Build history of the part. All positions in model axes, mm. A direction names the side the tool comes from. Coordinates: 2 decimals unless noted, no trailing zeros. Order: outer loops, then holes, each group sorted by start corner. A loop starts at its lowest first (then second) coordinate and runs counter-clockwise, first axis right, second up. Notation, with made-up numbers: (74, -29) - (90, -29) arc R35 cw to (90, 5) - close; hole circle Ø10 at (16, 10). An arc over 180 degrees is marked (long way). Write each question's results on one line, items separated by ' | '. Start each with the question number.
from build123d import *

# Parameters (mm, degrees)
SKETCH1_W              = 120
SKETCH1_H              = 250
BOSS_EXTRUDE2_DEPTH    = 100
CUT_EXTRUDE1_DEPTH     = 295.78805946
CUT_EXTRUDE3_START     = -120
CUT_EXTRUDE3_OUTLINE_R = 12.5
CUT_EXTRUDE3_DEPTH     = 120
CUT_EXTRUDE4_DEPTH     = 60
BOSS_EXTRUDE3_DEPTH    = 40


# Read off the part's stored shape, not the designer's step: Cut-Extrude3
with BuildPart() as part:
    # Sketch1 → Boss-Extrude2 (new body)
    with BuildSketch(Plane(origin=(0, 0, 0), x_dir=(1, 0, 0), z_dir=(0, 1, 0))):
        with Locations((-60, 125)):
            Rectangle(SKETCH1_W, SKETCH1_H)
    extrude(amount=BOSS_EXTRUDE2_DEPTH)

    # Sketch4 → Cut-Extrude1 (cut, through all)
    with BuildSketch(Plane(origin=(0, 100, 0), x_dir=(1, 0, 0), z_dir=(0, 1, 0))):
        with BuildLine():
            ThreePointArc((-30, 51.988343819), (-44.471725446, 45.999266659), (-60, 43.956579222))
            Line((-60, 43.956579222), (-60, 0))
            Line((-60, 0), (-30, 0))
            Line((-30, 0), (-30, 51.988343819))
        make_face()
        with BuildLine():
            Line((-60, 0), (-60, 43.956579222))
            ThreePointArc((-60, 43.956579222), (-75.528274554, 45.999266659), (-90, 51.988343819))
            Line((-90, 51.988343819), (-90, 0))
            Line((-90, 0), (-60, 0))
        make_face()
        with BuildLine():
            ThreePointArc((-30, 100), (-38.786796564, 121.213203436), (-60, 130))
            Line((-60, 130), (-60, 43.956579222))
            ThreePointArc((-60, 43.956579222), (-44.471725446, 45.999266659), (-30, 51.988343819))
            Line((-30, 51.988343819), (-30, 100))
        make_face()
        with BuildLine():
            Line((-60, 43.956579222), (-60, 130))
            ThreePointArc((-60, 130), (-81.213203436, 121.213203436), (-90, 100))
            Line((-90, 100), (-90, 51.988343819))
            ThreePointArc((-90, 51.988343819), (-75.528274554, 45.999266659), (-60, 43.956579222))
        make_face()
        with BuildLine():
            Line((0, 250), (-30, 250))
            Line((-30, 250), (-30, 179.561593793))
            ThreePointArc((-30, 179.561593793), (-26.46215881, 161.088158847), (-16.349288051, 145.228967063))
            ThreePointArc((-16.349288051, 145.228967063), (-4.636985506, 127.241105931), (0, 106.283063455))
            Line((0, 106.283063455), (0, 250))
        make_face()
        with BuildLine():
            Line((-90, 179.561593793), (-90, 250))
            Line((-90, 250), (-120, 250))
            Line((-120, 250), (-120, 106.283063455))
            ThreePointArc((-120, 106.283063455), (-115.363014494, 127.241105931), (-103.650711949, 145.228967063))
            ThreePointArc((-103.650711949, 145.228967063), (-93.53784119, 161.088158847), (-90, 179.561593793))
        make_face()
    extrude(amount=-CUT_EXTRUDE1_DEPTH, mode=Mode.SUBTRACT)

    # Cut-Extrude3 outline → Cut-Extrude3 (cut)
    with BuildSketch(Plane(origin=(0, 0, 0), x_dir=(0, 0, -1), z_dir=(1, 0, 0)).offset(CUT_EXTRUDE3_START)):
        with BuildLine():
            ThreePointArc((50.000000003, 100), (68.257418585, 96.547466812), (83.993463424, 86.666666667))
            ThreePointArc((83.993463424, 86.666666667), (91.861485844, 81.726266594), (100.990195136, 80))
            Line((100.990195136, 80), (250, 80))
            Line((250, 80), (250, 100))
            Line((250, 100), (50.000000003, 100))
        make_face()
        with BuildLine():
            ThreePointArc((0, 49.999999696), (14.644660835, 85.355338953), (50.000000003, 100))
            Line((50.000000003, 100), (0, 100))
            Line((0, 100), (0, 49.999999696))
        make_face()
        with BuildLine():
            ThreePointArc((50, 0), (14.644661048, 14.644660833), (0, 49.999999696))
            Line((0, 49.999999696), (0, 0))
            Line((0, 0), (50, 0))
        make_face()
        with BuildLine():
            ThreePointArc((83.993463424, 13.333333333), (68.257418584, 3.452533187), (50, 0))
            Line((50, 0), (250, 0))
            Line((250, 0), (250, 20))
            Line((250, 20), (100.990195136, 20))
            ThreePointArc((100.990195136, 20), (91.861485844, 18.273733406), (83.993463424, 13.333333333))
        make_face()
        with Locations((50, 50)):
            Circle(CUT_EXTRUDE3_OUTLINE_R)
    extrude(amount=CUT_EXTRUDE3_DEPTH, mode=Mode.SUBTRACT)

    # Sketch6 → Cut-Extrude4 (cut)
    with BuildSketch(Plane(origin=(0, 0, -250), x_dir=(-1, 0, 0), z_dir=(0, 0, -1))):
        Polygon((30, 63), (47, 80), (30, 80), align=None)
        Polygon((81.5, 71.5), (90, 80), (73, 80), align=None)
        Polygon((90, 63), (90, 80), (81.5, 71.5), align=None)
        Polygon((90, 20), (90, 37), (73, 20), align=None)
        Polygon((30, 20), (38.5, 28.5), (30, 37), align=None)
        Polygon((47, 20), (38.5, 28.5), (30, 20), align=None)
    extrude(amount=-CUT_EXTRUDE4_DEPTH, mode=Mode.SUBTRACT)

    # Sketch6_3 → Boss-Extrude3 (add)
    with BuildSketch(Plane(origin=(0, 0, -250), x_dir=(-1, 0, 0), z_dir=(0, 0, -1))):
        with BuildLine():
            ThreePointArc((85, 50), (83.096988313, 59.567085809), (77.67766953, 67.67766953))
            Line((77.67766953, 67.67766953), (42.32233047, 32.32233047))
            ThreePointArc((42.32233047, 32.32233047), (69.567085809, 26.903011687), (85, 50))
        make_face()
        with BuildLine():
            Line((42.32233047, 32.32233047), (77.67766953, 67.67766953))
            ThreePointArc((77.67766953, 67.67766953), (42.32233047, 67.67766953), (42.32233047, 32.32233047))
        make_face()
    extrude(amount=BOSS_EXTRUDE3_DEPTH)


solid = part.part
Item 1: Slice it at D-D (y = 7.5). Write the cut outline in (x, z).
Item 2: Pull direction X, two halves, no side cores. Call faces 5 (the cylindrical face through (-15.218, 81.774, -91.74)), 6 (the flat face through (-30, 40, -60)), 7 (the cylindrical face through (-26.559, 50.42, -161.335)): released by +X, released by -X, zero draft, split by the parting line, or undercut.
Item 3: Flat gauge pins, fed straight in: P1, Ø10, axis at x = -101, y = 46, coming from the -Z side; P2, Ø8.5, axis at x = -83, y = 28, coming from the -Z side; P3, Ø22.5, axis at y = 50, z = -50, coming from the +X side; P4, Ø6, axis at y = 17.5, z = -114.5, coming from the -X side. Where does each tip first touch, or does it go through?
Item 4: Slice it at C-C (x = -111). Write the cut outline in (y, z), then the cut area to 3 significant figures.
Item 5: Slice it at A-A (y = 45.5). Write the cut outline in (x, z).
Item 6: Which spindle directions (+Z, -Z, +X, -X, +Y, -Y) get a long thin tool onto all of the face, cutting with end or side? Do faces 1 (the flat face through (-85, 25, -190)), 2 (the flat face through (-35, 25, -190)), 3 (the flat face through (-90, 40, -40)), 4 (the flat face through (-85, 45, -250)). Say none if no direction does.
Item 7: Slice it at B-B (z = -92). Write the cut outline in (x, y), then the cut area to 3 significant figures.
Item 8: Probe probe 1 along X at (y, z) = (36, -100); probe 2 along Y at (x, z) = (-102, -50); probe 3 along Y at (x, z) = (-5, -106). List the from-to ranges inside material, lowest first.
Resolved:
1) outline: (-120, -76.34) - (-90, -76.34) - (-90, -23.66) - (-120, -23.66) - close; (-30, -76.34) - (0, -76.34) - (0, -23.66) - (-30, -23.66) - close
2) face 5: zero draft | face 6: undercut | face 7: released by +X
3) P1: z = -155.81 | P2: z = -250 | P3: through | P4: x = -119.39
4) outline: (13.33, -83.99) arc R25 cw to (20, -100.99) - (20, -135.69) - (80, -135.69) - (80, -100.99) arc R25 cw to (86.67, -83.99) arc R50 ccw (long way) to start; hole circle Ø25 at (50, -50) | area: 9,720 mm^2
5) outline: (-120, -106.28) arc R60.04 ccw to (-103.65, -145.23) arc R50 cw to (-90, -179.56) - (-90, -250) - (-84.59, -250) - (-84.59, -290) - (-35.41, -290) - (-35.41, -250) - (-30, -250) - (-30, -179.56) arc R50 cw to (-16.35, -145.23) arc R60.04 ccw to (0, -106.28) - (0, -61.66) - (-30, -61.66) - (-30, -100) arc R30 cw to (-90, -100) - (-90, -61.66) - (-120, -61.66) - close; (-120, -38.34) - (-90, -38.34) - (-90, -0.2) - (-120, -0.2) - close; (-30, -38.34) - (0, -38.34) - (0, -0.2) - (-30, -0.2) - close
6) face 1: -Z, -X, -Y | face 2: -Z, +X, -Y | face 3: +Z, +Y, -Y | face 4: -Z
7) outline: (-120, 18.33) - (-90, 18.33) - (-90, 81.67) - (-120, 81.67) - close; (-30, 18.33) - (0, 18.33) - (0, 81.67) - (-30, 81.67) - close | area: 3,800 mm^2
8) probe 1: -120 to -90, -30 to 0 | probe 2: 0 to 37.5, 62.5 to 100 | probe 3: 20 to 80
